Could you check a few things on this model? Use its own coordinates, in mm. A direction names the side the tool comes from. Give positions to 0.01 mm unless a question says otherwise; leave off trailing zeros. Loops run counter-clockwise (first coordinate to the right, second up) from the corner with the lowest first, then second, coordinate; pieces in that order, holes last. Notation, with made-up numbers: M 7,-13.5 L 38,-13.5 A14 cw 38,11.5 Z; hole C 19,71 d1. An arc over 180 degrees is marked long. Answer in a Markdown table with one row per item. Add a question column.
```python
from build123d import *

# Parameters (mm, degrees)
SKETCH_1_W          = 20
SKETCH_1_H          = 10
SKETCH_1_W_2        = 17
SKETCH_1_H_2        = 7
EXTRUDE_1_DEPTH     = 114.5
SKETCH_2_R          = 2.1
CUT_EXTRUDE_1_DEPTH = 117.341093342
SKETCH_3_R          = 2.1
CUT_EXTRUDE_2_DEPTH = 117.341093342
SKETCH_4_R          = 2.1
CUT_EXTRUDE_3_DEPTH = 116.370056774


with BuildPart() as part:
    # ｽｹｯﾁ1 → 押し出し-薄板1 (new body)
    with BuildSketch(Plane.XY):
        Rectangle(SKETCH_1_W, SKETCH_1_H)
        Rectangle(SKETCH_1_W_2, SKETCH_1_H_2, mode=Mode.SUBTRACT)
    extrude(amount=EXTRUDE_1_DEPTH)

    # ｽｹｯﾁ2 → ｶｯﾄ - 押し出し1 (cut, through all)
    with BuildSketch(Plane(origin=(10, 0, 0), x_dir=(0, 0, -1), z_dir=(1, 0, 0))):
        with Locations(Location((-97, 0, 0), (0, 0, 90))):
            Circle(SKETCH_2_R)
        with Locations(Location((-32, 0, 0), (0, 0, 90))):
            Circle(SKETCH_2_R)
    extrude(amount=-CUT_EXTRUDE_1_DEPTH, mode=Mode.SUBTRACT)

    # ｽｹｯﾁ3 → ｶｯﾄ - 押し出し2 (cut, through all)
    with BuildSketch(Plane(origin=(10, 0, 0), x_dir=(0, 0, -1), z_dir=(1, 0, 0))):
        with Locations(Location((-5, 0, 0), (0, 0, 90))):
            Circle(SKETCH_3_R)
    extrude(amount=-CUT_EXTRUDE_2_DEPTH, mode=Mode.SUBTRACT)

    # ｽｹｯﾁ4 → ｶｯﾄ - 押し出し3 (cut, through all)
    with BuildSketch(Plane(origin=(0, 5, 0), x_dir=(1, 0, 0), z_dir=(0, 1, 0))):
        with Locations(Location((0, -19.5, 0), (0, 0, 270))):
            Circle(SKETCH_4_R)
        with Locations(Location((0, -109.5, 0), (0, 0, 270))):
            Circle(SKETCH_4_R)
    extrude(amount=-CUT_EXTRUDE_3_DEPTH, mode=Mode.SUBTRACT)


solid = part.part
```
Item 1: Suppose I cut it at D-D (z = 13). List the corners of the cut face in (x, y) for me, then the cut area to 3 significant figures.
Item 2: Suppose I cut it at C-C (x = 0). List the corners of the cut face in (y, z) for me.
Item 3: For P1, Ø4, axis at y = 0, z = 97, coming from the +X side, with a flat end and sliding along its axis, tell me the tip position at first contact or that it passes through.
Item 4: Suppose I cut it at A-A (y = 0). Give the number of separate pieces and of enclosed holes in the cut face, then the cut area to 3 significant figures.
Item 5: I need wall thicknesses on L1, parallel to Z at x = -8.75, y = 0; L2, parallel to X at y = -3.95, z = 19.5; L3, parallel to X at y = -2.5, z = 17. Which ranges of each line are inside material? Lowest first, please.
Item 6: If we mould it in two halves opening along Y, with no side actions, what happens to faces 1 (the face through (0, 5, 56)), 2 (the face through (8.5, 0, 56)), 3 (the face through (0, -4, 0))? For each: +Y half, -Y half, draft (parallel to the pull), parting line (faces both ways), or undercut.
Item 7: Suppose I cut it at B-B (z = 109.5). List the corners of the cut face in (x, y) for me, then the cut area to 3 significant figures.
Item 8: For faces 4 (the face through (0, 3.5, 56)), 5 (the face through (0, -4, 114.5)), which set-ups out of +Z, -Z, +X, -X, +Y, -Y let a thin tool reach every point of the face, with its end or its side?
Values found:
| question | item | result |
|---|---|---|
| 1 | outline | M -10,-5 L 10,-5 L 10,5 L -10,5 Z; hole M -8.5,-3.5 L 8.5,-3.5 L 8.5,3.5 L -8.5,3.5 Z |
| 1 | area | 81.0 mm² |
| 2 | outline | M -5,0 L -3.5,0 L -3.5,17.4 L -5,17.4 Z; M -5,21.6 L -3.5,21.6 L -3.5,107.4 L -5,107.4 Z; M -5,111.6 L -3.5,111.6 L -3.5,114.5 L -5,114.5 Z; M 3.5,0 L 5,0 L 5,17.4 L 3.5,17.4 Z; M 3.5,21.6 L 5,21.6 L 5,107.4 L 3.5,107.4 Z; M 3.5,111.6 L 5,111.6 L 5,114.5 L 3.5,114.5 Z |
| 3 | P1 | through |
| 4 | separate pieces | 8 |
| 4 | enclosed holes | 0 |
| 4 | area | 306 mm² |
| 5 | L1 | 0 to 2.9, 7.1 to 29.9, 34.1 to 94.9, 99.1 to 114.5 |
| 5 | L2 | -10 to -2.1, 2.1 to 10 |
| 5 | L3 | -10 to -8.5, 8.5 to 10 |
| 6 | face 1 | +Y half |
| 6 | face 2 | undercut |
| 6 | face 3 | draft |
| 7 | outline | M -10,-5 L -2.1,-5 L -2.1,-3.5 L -8.5,-3.5 L -8.5,3.5 L -2.1,3.5 L -2.1,5 L -10,5 Z; M 2.1,-5 L 10,-5 L 10,5 L 2.1,5 L 2.1,3.5 L 8.5,3.5 L 8.5,-3.5 L 2.1,-3.5 Z |
| 7 | area | 68.4 mm² |
| 8 | face 4 | +Z, -Z |
| 8 | face 5 | +Z, +X, -X, +Y, -Y |
